Part model, mm, in its own coordinate system. A direction names the side the tool comes from. Round coordinates to 2 decimals unless told otherwise and drop trailing zeros. Loops run counter-clockwise (first coordinate to the right, second up) from the corner with the lowest first, then second, coordinate; pieces in that order, holes last. Notation, with made-up numbers: (85.25, 4) - (101.25, 4) arc R27 cw to (101.25, 25) - close; hole circle Ø11 at (-23.75, -6). An arc over 180 degrees is marked (long way). Write each question's results on one line, items separated by ' | '. Start each with the question number.
(1) Cut at D-D, the plane x = 0. List the corners of the cut face in (y, z).
(2) Cut at A-A, the plane x = 5.5. List the corners of the cut face in (y, z), then the cut area to 3 significant figures.
(3) Cut at B-B, the plane z = 7. List the corners of the cut face in (x, y), then the cut area to 4 significant figures.
(4) Drill centre lines: L1, parallel to Y at x = 3.5, z = -5.25; L2, parallel to X at y = 5.25, z = -3; L3, parallel to Y at x = -4, z = -3.25. Where is each one in solid material? Low to high.
(5) Tool access for faces 1 (the face through (-5.862, 5, 2)), 2 (the face through (7.888, 5, 2)), 3 (the face through (1, 8.5, 6)), 4 (the face through (1, 5, -3.565)), 5 (the face through (1, 5, 7.435)): list every direction of +Z, -Z, +X, -X, +Y, -Y with a clear straight run to the whole face (end or side of a thin tool).
(6) Cut at C-C, the plane y = 5.5. List the corners of the cut face in (x, z).
(7) Flat gauge pins, fed straight in: P1, Ø6, axis at x = 8, z = -1, coming from the +Y side; P2, Ø5, axis at y = 8.5, z = 6, coming from the +X side; P3, Ø8, axis at y = 13, z = 7.5, coming from the -X side. Where does each tip first touch, or does it go through?
from build123d import *

# Parameters (mm, degrees)
SKETCH1_W           = 33.5
SKETCH1_H           = 20
BOSS_EXTRUDE1_DEPTH = 1.5
SKETCH2_W           = 13.75
SKETCH2_H           = 11
BOSS_EXTRUDE2_DEPTH = 7
SKETCH3_R           = 3.5
BOSS_EXTRUDE3_DEPTH = 7
SKETCH4_R           = 3
BOSS_EXTRUDE4_DEPTH = 13
CUT_EXTRUDE1_START  = -10
CUT_EXTRUDE1_DEPTH  = 10


with BuildPart() as part:
    # Sketch1 → Boss-Extrude1 (new body)
    with BuildSketch(Plane(origin=(0, 0, 0), x_dir=(1, 0, 0), z_dir=(0, 1, 0))):
        with Locations((7.887566138, -1.935185185)):
            Rectangle(SKETCH1_W, SKETCH1_H)
    extrude(amount=BOSS_EXTRUDE1_DEPTH)

    # Sketch2 → Boss-Extrude2 (add)
    with BuildSketch(Plane(origin=(0, 1.5, 0), x_dir=(1, 0, 0), z_dir=(0, 1, 0))):
        with Locations((1.012566138, -1.935185185)):
            Rectangle(SKETCH2_W, SKETCH2_H)
    extrude(amount=BOSS_EXTRUDE2_DEPTH)

    # Sketch3 → Boss-Extrude3 (add)
    with BuildSketch(Plane(origin=(0, 8.5, 0), x_dir=(1, 0, 0), z_dir=(0, 1, 0))):
        with Locations(Location((1.137566138, -1.784110138, 0), (0, 0, 270))):
            Circle(SKETCH3_R)
    extrude(amount=BOSS_EXTRUDE3_DEPTH)

    # Sketch4 → Boss-Extrude4 (add)
    with BuildSketch(Plane(origin=(0, 15.5, 0), x_dir=(1, 0, 0), z_dir=(0, 1, 0))):
        with Locations(Location((1.137566138, -1.784110138, 0), (0, 0, 90))):
            Circle(SKETCH4_R)
    extrude(amount=BOSS_EXTRUDE4_DEPTH)

    # Sketch5 → Cut-Extrude1 (cut)
    with BuildSketch(Plane(origin=(0, 28.5, 0), x_dir=(1, 0, 0), z_dir=(0, 1, 0)).offset(CUT_EXTRUDE1_START)):
        with BuildLine():
            Line((2.637566138, -1.784110138), (2.637566138, 0.813966073))
            ThreePointArc((2.637566138, 0.813966073), (4.137566138, -1.784110138), (2.637566138, -4.382186349))
            Line((2.637566138, -4.382186349), (2.637566138, -1.784110138))
        make_face()
    extrude(amount=CUT_EXTRUDE1_DEPTH, mode=Mode.SUBTRACT)


solid = part.part
A:
1) outline: (0, -8.06) - (1.5, -8.06) - (1.5, -3.56) - (8.5, -3.56) - (8.5, -1.53) - (15.5, -1.53) - (15.5, -0.99) - (28.5, -0.99) - (28.5, 4.56) - (15.5, 4.56) - (15.5, 5.09) - (8.5, 5.09) - (8.5, 7.44) - (1.5, 7.44) - (1.5, 11.94) - (0, 11.94) - close
2) outline: (0, -8.06) - (1.5, -8.06) - (1.5, -3.56) - (8.5, -3.56) - (8.5, 7.44) - (1.5, 7.44) - (1.5, 11.94) - (0, 11.94) - close | area: 107 mm2
3) outline: (-8.86, 0) - (24.64, 0) - (24.64, 1.5) - (7.89, 1.5) - (7.89, 8.5) - (-5.86, 8.5) - (-5.86, 1.5) - (-8.86, 1.5) - close | area: 146.5 mm2
4) L1: 0 to 1.5 | L2: -5.86 to 7.89 | L3: 0 to 8.5
5) face 1: +Z, -Z, -X, +Y | face 2: +Z, -Z, +X, +Y | face 3: +Y | face 4: -Z, +X, -X, +Y | face 5: +Z, +X, -X, +Y
6) outline: (-5.86, -3.56) - (7.89, -3.56) - (7.89, 7.44) - (-5.86, 7.44) - close
7) P1: y = 8.5 | P2: x = 7.89 | P3: x = -1.91
